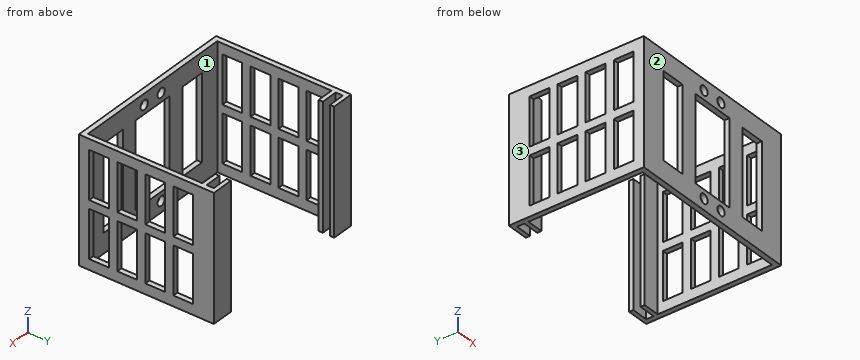
```python
from build123d import *

# Parameters (mm, degrees)
PAD_DEPTH       = 60
SKETCH_R        = 2.25
SKETCH_W        = 12
SKETCH_H        = 41
POCKET_DEPTH    = 3
SKETCH002_W     = 9.5
SKETCH002_H     = 23
POCKET001_DEPTH = 85.001


with BuildPart() as part:
    # Sketch001 → Pad (new body)
    with BuildSketch(Plane(origin=(0, 0, 0), x_dir=(-1, 0, 0), z_dir=(0, 0, 1))):
        Polygon((-42.5, 0), (-42.5, -65), (-32, -65), (-32, -63), (-40, -63), (-40, -59.5), (-32, -59.5), (-32, -57.5), (-40, -57.5), (-40, -2.5), (0, -2.5), (40, -2.5), (40, -57.5), (32, -57.5), (32, -59.5), (40, -59.5), (40, -63), (32, -63), (32, -65), (42.5, -65), (42.5, 0), align=None)
    extrude(amount=PAD_DEPTH)

    # Sketch (on Face1 of Pad) → Pocket (cut)
    with BuildSketch(Plane(origin=(0, 0, 30), x_dir=(1, 0, 0), z_dir=(0, -1, 0))):
        with Locations((-5.25, 24.75)):
            Circle(SKETCH_R)
        with Locations((-5.25, -24.75)):
            Circle(SKETCH_R)
        with Locations((5.25, -24.75)):
            Circle(SKETCH_R)
        with Locations((5.25, 24.75)):
            Circle(SKETCH_R)
        Polygon((10.5, 20.5), (10.5, -20.5), (-10.5, -20.5), (-10.5, 0), (-10.5, 20.5), (0, 20.5), align=None)
        with Locations((-24.5, 0)):
            Rectangle(SKETCH_W, SKETCH_H)
        with Locations((24.5, 0)):
            Rectangle(SKETCH_W, SKETCH_H)
    extrude(amount=-POCKET_DEPTH, mode=Mode.SUBTRACT)

    # Sketch002 (on Face5 of Pocket) → Pocket001 (cut, through all)
    with BuildSketch(Plane(origin=(-42.5, 0, 0), x_dir=(0, -1, 0), z_dir=(-1, 0, 0))):
        with Locations((-9.75, 16.5)):
            Rectangle(SKETCH002_W, SKETCH002_H)
        with Locations((-23.25, 16.5)):
            Rectangle(SKETCH002_W, SKETCH002_H)
        with Locations((-9.75, 43.5)):
            Rectangle(SKETCH002_W, SKETCH002_H)
        with Locations((-23.25, 43.5)):
            Rectangle(SKETCH002_W, SKETCH002_H)
        with Locations((-36.75, 43.5)):
            Rectangle(SKETCH002_W, SKETCH002_H)
        with Locations((-50.25, 43.5)):
            Rectangle(SKETCH002_W, SKETCH002_H)
        with Locations((-36.75, 16.5)):
            Rectangle(SKETCH002_W, SKETCH002_H)
        with Locations((-50.25, 16.5)):
            Rectangle(SKETCH002_W, SKETCH002_H)
    extrude(amount=-POCKET001_DEPTH, mode=Mode.SUBTRACT)


solid = part.part
```
Geometry check sheet. Reference: the model listing, model coordinates, mm. Face numbers are marked on the shaded views. Give positions to 0.01 mm unless a question says otherwise; leave off trailing zeros. Order: outer loops, then holes, each group sorted by start corner. A loop starts at its lowest first (then second) coordinate and runs counter-clockwise, first axis right, second up. Notation, with made-up numbers: (23.25, 42) -> (41.25, 42) arc R20 cw to (41.25, 79) -> close; hole circle Ø8 at (31.25, -30). An arc over 180 degrees is marked (long way). Write each question's results on one line, items separated by ' | '. Start each with the question number.
(1) Gauge pin test, flat end, axial feed: P1, Ø4, axis at x = -14, z = 51, coming from the +Y side. Record the tip position at first contact, or that the pin passes through.
(2) Sectioned sample at B-B (x = 5.25). Enter the section's corners in (y, z), plus the area to 3 significant figures.
(3) Sectioned sample at A-A (y = 40). Enter the section's corners in (x, z), plus the area to 3 significant figures.
(4) Sectioned sample at D-D (y = 29.5). Enter the section's corners in (x, z), plus the area to 3 significant figures.
(5) Mould release check, pull along Y, two halves, no side actions. Record for the marked faces 1, 2 and 3: pulls with the +Y half, pulls with the -Y half, needs draft (parallel to the pull), parting line crosses it, or undercut.
(6) Scan lines: line 1 (Z direction, x = 5, y = 1); line 2 (Y direction, x = 37, z = 14.5); line 3 (X direction, y = 29, z = 11). Record each from-to range of solid material in increasing order.
(7) Sectioned sample at C-C (x = 25). Enter the section's corners in (y, z), plus the area to 3 significant figures.
Answer below:
1) P1: y = 2.5
2) outline: (0, 0) -> (2.5, 0) -> (2.5, 3) -> (0, 3) -> close; (0, 7.5) -> (2.5, 7.5) -> (2.5, 9.5) -> (0, 9.5) -> close; (0, 50.5) -> (2.5, 50.5) -> (2.5, 52.5) -> (0, 52.5) -> close; (0, 57) -> (2.5, 57) -> (2.5, 60) -> (0, 60) -> close | area: 25.0 mm2
3) outline: (-42.5, 0) -> (-40, 0) -> (-40, 5) -> (-42.5, 5) -> close; (-42.5, 28) -> (-40, 28) -> (-40, 32) -> (-42.5, 32) -> close; (-42.5, 55) -> (-40, 55) -> (-40, 60) -> (-42.5, 60) -> close; (40, 0) -> (42.5, 0) -> (42.5, 5) -> (40, 5) -> close; (40, 28) -> (42.5, 28) -> (42.5, 32) -> (40, 32) -> close; (40, 55) -> (42.5, 55) -> (42.5, 60) -> (40, 60) -> close | area: 70.0 mm2
4) outline: (-42.5, 0) -> (-40, 0) -> (-40, 60) -> (-42.5, 60) -> close; (40, 0) -> (42.5, 0) -> (42.5, 60) -> (40, 60) -> close | area: 300 mm2
5) face 1: undercut | face 2: pulls with the -Y half | face 3: needs draft
6) line 1: 0 to 3.01, 7.49 to 9.5, 50.5 to 52.51, 56.99 to 60 | line 2: 0 to 2.5, 57.5 to 59.5, 63 to 65 | line 3: -42.5 to -40, 40 to 42.5
7) outline: (0, 0) -> (2.5, 0) -> (2.5, 9.5) -> (0, 9.5) -> close; (0, 50.5) -> (2.5, 50.5) -> (2.5, 60) -> (0, 60) -> close | area: 47.5 mm2
